from build123d import *

# Parameters (mm, degrees)
F0_R     = 64.2875
F0_R_2   = 14.2875
F1_DEPTH = 3.175
F3_DEPTH = 25


with BuildPart() as f1:
    # F0 (on Top) → F1 (new body)
    with BuildSketch(Plane.XY):
        Circle(F0_R)
        Circle(F0_R_2, mode=Mode.SUBTRACT)
    extrude(amount=F1_DEPTH)

    # F2 (on face) → F3 (cut)
    with BuildSketch(Plane.XY.offset(3.175)):
        with BuildLine():
            ThreePointArc((-40, 35), (-36.464466, 36.464466), (-35, 40))
            Line((-35, 40), (-40, 40))
            Line((-40, 40), (-40, 35))
        make_face()
        with BuildLine():
            Line((-40, 40), (-35, 40))
            ThreePointArc((-35, 40), (-43.535534, 43.535534), (-40, 35))
            Line((-40, 35), (-40, 40))
        make_face()
        with BuildLine():
            Line((40, 40), (35, 40))
            ThreePointArc((35, 40), (36.464466, 36.464466), (40, 35))
            Line((40, 35), (40, 40))
        make_face()
        with BuildLine():
            ThreePointArc((45, 40), (40, 45), (35, 40))
            Line((35, 40), (40, 40))
            Line((40, 40), (40, 35))
            ThreePointArc((40, 35), (43.535534, 36.464466), (45, 40))
        make_face()
        with BuildLine():
            ThreePointArc((45, -40), (43.535534, -36.464466), (40, -35))
            Line((40, -35), (40, -40))
            Line((40, -40), (35, -40))
            ThreePointArc((35, -40), (40, -45), (45, -40))
        make_face()
        with BuildLine():
            Line((40, -40), (40, -35))
            ThreePointArc((40, -35), (36.464466, -36.464466), (35, -40))
            Line((35, -40), (40, -40))
        make_face()
        with BuildLine():
            Line((-40, -40), (-40, -35))
            ThreePointArc((-40, -35), (-43.535534, -43.535534), (-35, -40))
            Line((-35, -40), (-40, -40))
        make_face()
        with BuildLine():
            ThreePointArc((-35, -40), (-36.464466, -36.464466), (-40, -35))
            Line((-40, -35), (-40, -40))
            Line((-40, -40), (-35, -40))
        make_face()
    extrude(amount=-F3_DEPTH, mode=Mode.SUBTRACT)


solid = f1.part
Verification items for the finished model (mm, model axes). Give positions to 0.01 mm unless a question says otherwise; leave off trailing zeros. Write each loop counter-clockwise with the first axis right and the second up, starting at its lowest first coordinate (ties: lowest second). Pieces come first, ordered by that corner, then holes. Notation, with made-up numbers: (66, 49) - (108, 49) arc R19 ccw to (108, 75) - close; hole circle Ø1 at (23, 59). An arc over 180 degrees is marked (long way). Answer as CSV lines item,"result". Start each with the question number.
1. Sectioned sample at A-A (x = 0). Record the boundary of the cut face in (y, z) (1 decimal), then the cut area to 4 significant figures.
2. Sectioned sample at D-D (y = -17). Record the boundary of the cut face in (x, z) (3 decimals), then the cut area to 3 significant figures.
3. Thickness scan on line 1 (Y direction, x = 1, z = 2.8); line 2 (Y direction, x = -40, z = 1.8). Record the ranges inside material, lowest first.
4. Draft check along X on faces 1 (the face through (-1, 15, 0)), 2 (the face through (-14.274, 0.628, 1.565)), 3 (the face through (-13.936, -62.759, 1.565)). Enter one of: pulls with the +X half, pulls with the -X half, needs draft (parallel to the pull), parting line crosses it, or undercut.
5. Sectioned sample at C-C (z = 2.25). Record the boundary of the cut face in (x, y) (1 decimal).
Derived:
1,outline,"(-64.3, 0) - (-14.3, 0) - (-14.3, 3.2) - (-64.3, 3.2) - close; (14.3, 0) - (64.3, 0) - (64.3, 3.2) - (14.3, 3.2) - close"
1,area,"317.5 mm²"
2,outline,"(-61.999, 0) - (61.999, 0) - (61.999, 3.175) - (-61.999, 3.175) - close"
2,area,"394 mm²"
3,line 1,"-64.28 to -14.25, 14.25 to 64.28"
3,line 2,"-50.33 to -45, -35 to 35, 45 to 50.33"
4,face 1,"needs draft"
4,face 2,"undercut"
4,face 3,"parting line crosses it"
5,outline,"circle Ø128.6 at (0, 0); hole circle Ø10 at (-40, -40); hole circle Ø10 at (-40, 40); hole circle Ø28.6 at (0, 0); hole circle Ø10 at (40, -40); hole circle Ø10 at (40, 40)"
